```python
from build123d import *

# Parameters (mm, degrees)
F1_DEPTH = 6.35
F4_D     = 3.9878


with BuildPart() as f1:
    # F0 (on Front) → F1 (new body)
    with BuildSketch(Plane.XZ):
        with BuildLine():
            ThreePointArc((-2.078402, 2.400181), (-1.600052, 2.742345), (-1.0668, 2.990412))
            Line((-1.0668, 2.990412), (-1.0668, 4.192946))
            Line((-1.0668, 4.192946), (-1.0668, 8.750181))
            Line((-1.0668, 8.750181), (-2.078402, 8.750181))
            Line((-2.078402, 8.750181), (-2.078402, 4.192946))
            Line((-2.078402, 4.192946), (-2.078402, 2.400181))
        make_face()
        with BuildLine():
            ThreePointArc((1.0668, 1.175625), (0, -1.5875), (-1.0668, 1.175625))
            Line((-1.0668, 1.175625), (-1.0668, 2.990412))
            ThreePointArc((-1.0668, 2.990412), (-1.600052, 2.742345), (-2.078402, 2.400181))
            ThreePointArc((-2.078402, 2.400181), (-3.12438, 0.564687), (-2.787067, -1.520817))
            ThreePointArc((-2.787067, -1.520817), (-2.194353, -2.294655), (-1.394812, -2.852214))
            Line((-1.394812, -2.852214), (1.394812, -2.852214))
            ThreePointArc((1.394812, -2.852214), (2.194353, -2.294655), (2.787067, -1.520817))
            ThreePointArc((2.787067, -1.520817), (3.12438, 0.564687), (2.078402, 2.400181))
            ThreePointArc((2.078402, 2.400181), (1.600052, 2.742345), (1.0668, 2.990412))
            Line((1.0668, 2.990412), (1.0668, 1.175625))
        make_face()
        with BuildLine():
            Line((1.0668, 4.192946), (1.0668, 2.990412))
            ThreePointArc((1.0668, 2.990412), (1.600052, 2.742345), (2.078402, 2.400181))
            Line((2.078402, 2.400181), (2.078402, 4.192946))
            Line((2.078402, 4.192946), (2.078402, 8.750181))
            Line((2.078402, 8.750181), (1.0668, 8.750181))
            Line((1.0668, 8.750181), (1.0668, 4.192946))
        make_face()
        with BuildLine():
            Line((14.078129, -1.520817), (2.787067, -1.520817))
            ThreePointArc((2.787067, -1.520817), (2.194353, -2.294655), (1.394812, -2.852214))
            Line((1.394812, -2.852214), (14.078129, -2.852214))
            Line((14.078129, -2.852214), (14.078129, -1.520817))
        make_face()
        with BuildLine():
            ThreePointArc((-1.394812, -2.852214), (-2.194353, -2.294655), (-2.787067, -1.520817))
            Line((-2.787067, -1.520817), (-14.078129, -1.520817))
            Line((-14.078129, -1.520817), (-14.078129, -2.852214))
            Line((-14.078129, -2.852214), (-1.394812, -2.852214))
        make_face()
    extrude(amount=F1_DEPTH)

    # F4 (through all)
    with Locations(Plane(origin=(0, 0, -2.852214), x_dir=(1, 0, 0), z_dir=(0, 0, -1))):
        with Locations((-8.219072, 3.175), (8.219072, 3.175)):
            Hole(F4_D / 2)


solid = f1.part
```
Model file for the job. Use its own axes, mm. A direction names the side the tool comes from. Give positions to 0.01 mm unless a question says otherwise; leave off trailing zeros. Loops run counter-clockwise (first coordinate to the right, second up) from the corner with the lowest first, then second, coordinate; pieces in that order, holes last. Notation, with made-up numbers: (39.5, 71) -> (55.5, 71) arc R16 ccw to (55.5, 99) -> close; hole circle Ø6 at (86.5, 49). An arc over 180 degrees is marked (long way). Use CSV: the item, a comma, the result in double quotes. Start each with the question number.
1) Tool access for faces 4 (the flat face through (14.078, -3, -2)), 5 (the flat face through (2.078, -3, 6)), 6 (the flat face through (1.067, -3, 5)): list every direction of +Z, -Z, +X, -X, +Y, -Y with a clear straight run to the whole face (end or side of a thin tool).
2) Wall check: line 1 (X direction, y = -3, z = 6.75); line 2 (X direction, y = -6, z = 0) (1 decimal); line 3 (Z direction, x = 11.5, y = -2). Give the ranges that are in metal, low to high.
3) Slice it at A-A on z = 3.75. Give the cut face in (x, y), plus the area to 3 significant figures.
4) Slice it at C-C on y = -4.75. Give the number of separate pieces and of enclosed holes in the cut face, plus the area to 3 significant figures.
5) Mould opens along X. For faces 1 (the flat face through (-1.067, -3, 5)), 2 (the flat face through (-2.078, -3, 6)), 3 (the flat face through (-1.6, -3.1, 8.75)) say: released by +X, released by -X, zero draft, split by the parting line, or undercut.
6) Slice it at D-D on x = -4. Give the cut face in (y, z).
7) Flat gauge pins, fed straight in: pin 1 Ø1.9 at (x, y) = (-10.5, -3.5) entering from +Z; pin 2 Ø3 at (y, z) = (-2.5, 5.5) entering from -X; pin 3 Ø1 at (y, z) = (-3, 0.5) entering from +X (3 decimals); pin 4 Ø2.5 at (x, y) = (8.22, -3.18) entering from -Z. Where does each tip first touch, or does it go through?
Computed values:
1,face 4,"+Z, -Z, +X, +Y, -Y"
1,face 5,"+Z, +X, +Y, -Y"
1,face 6,"+Z, +Y, -Y"
2,line 1,"x = -2.08 to -1.07, 1.07 to 2.08"
2,line 2,"x = -3.2 to -1.6, 1.6 to 3.2"
2,line 3,"z = -2.85 to -1.52"
3,outline,"(-2.08, -6.35) -> (-1.07, -6.35) -> (-1.07, 0) -> (-2.08, 0) -> close; (1.07, -6.35) -> (2.08, -6.35) -> (2.08, 0) -> (1.07, 0) -> close"
3,area,"12.8 mm^2"
4,separate pieces,"3"
4,enclosed holes,"0"
4,area,"56.8 mm^2"
5,face 1,"undercut"
5,face 2,"released by -X"
5,face 3,"zero draft"
6,outline,"(-6.35, -2.85) -> (0, -2.85) -> (0, -1.52) -> (-6.35, -1.52) -> close"
7,pin 1,"stops at z = -1.52"
7,pin 2,"stops at x = -2.08"
7,pin 3,"stops at x = 3.175"
7,pin 4,"passes through"
